from build123d import *

# Parameters (mm, degrees)
BOSS_EXTRUDE1_DEPTH = 21.59
SKETCH2_W           = 22.352
SKETCH2_H           = 21.6154
SKETCH2_R           = 3.175
BOSS_EXTRUDE2_DEPTH = 3.81
SKETCH3_R           = 3.175
BOSS_EXTRUDE3_DEPTH = 6.35
SKETCH4_W           = 27.94
SKETCH4_H           = 144.78
BOSS_EXTRUDE4_DEPTH = 48.388036719
SKETCH5_W           = 38.1
SKETCH5_H           = 30.48
SKETCH5_W_2         = 60.96
CUT_EXTRUDE1_DEPTH  = 385.104870976
SKETCH6_R           = 3.175
CUT_EXTRUDE2_DEPTH  = 833.884500924


with BuildPart() as part:
    # Sketch1 → Boss-Extrude1 (new body)
    with BuildSketch(Plane.XY):
        with BuildLine():
            Line((-792.583825879, 352.959436719), (-792.583825879, 356.769436719))
            Line((-792.583825879, 356.769436719), (-801.338321143, 356.769436719))
            ThreePointArc((-801.338321143, 356.769436719), (-803.772947911, 357.085841957), (-806.045825879, 358.014036719))
            ThreePointArc((-806.045825879, 358.014036719), (-810.863321143, 366.294436719), (-806.045825879, 374.574836719))
            Line((-806.045825879, 374.574836719), (-814.935825879, 374.574836719))
            Line((-814.935825879, 374.574836719), (-814.935825879, 352.959436719))
            Line((-814.935825879, 352.959436719), (-792.583825879, 352.959436719))
        make_face()
    extrude(amount=-BOSS_EXTRUDE1_DEPTH)

    # Sketch2 → Boss-Extrude2 (add)
    with BuildSketch(Plane.XY):
        with Locations((-803.759825879, 363.767136719)):
            Rectangle(SKETCH2_W, SKETCH2_H)
        with Locations(Location((-801.338321143, 366.294436719, 0), (0, 0, 180))):
            Circle(SKETCH2_R, mode=Mode.SUBTRACT)
    extrude(amount=BOSS_EXTRUDE2_DEPTH)

    # Sketch3 → Boss-Extrude3 (add)
    with BuildSketch(Plane(origin=(0, 0, -21.59), x_dir=(-1, 0, 0), z_dir=(0, 0, -1))):
        with BuildLine():
            Line((792.583825879, 356.769436719), (792.583825879, 374.574836719))
            Line((792.583825879, 374.574836719), (806.045825879, 374.574836719))
            ThreePointArc((806.045825879, 374.574836719), (810.546915906, 363.859809951), (801.338321143, 356.769436719))
            Line((801.338321143, 356.769436719), (792.583825879, 356.769436719))
        make_face()
        with Locations((801.338321143, 366.294436719)):
            Circle(SKETCH3_R, mode=Mode.SUBTRACT)
    extrude(amount=-BOSS_EXTRUDE3_DEPTH)

    # Sketch4 → Boss-Extrude4 (add)
    with BuildSketch(Plane.XZ.offset(-352.959436719)):
        with Locations((-813.665825879, 5.08)):
            Rectangle(SKETCH4_W, SKETCH4_H)
    extrude(amount=BOSS_EXTRUDE4_DEPTH)

    # Sketch5 → Cut-Extrude1 (cut, through all)
    with BuildSketch(Plane.ZY.offset(827.635825879)):
        with Locations((-48.26, 337.719436719)):
            Rectangle(SKETCH5_W, SKETCH5_H)
        with Locations((46.99, 337.719436719)):
            Rectangle(SKETCH5_W_2, SKETCH5_H)
    extrude(amount=-CUT_EXTRUDE1_DEPTH, mode=Mode.SUBTRACT)

    # Sketch6 → Cut-Extrude2 (cut, through all)
    with BuildSketch(Plane(origin=(0, 322.479436719, 0), x_dir=(1, 0, 0), z_dir=(0, 1, 0))):
        with Locations(Location((-820.039, 56.765714286, 0), (0, 0, 270))):
            Circle(SKETCH6_R)
        with Locations(Location((-820.039, -61.162857143, 0), (0, 0, 270))):
            Circle(SKETCH6_R)
    extrude(amount=-CUT_EXTRUDE2_DEPTH, mode=Mode.SUBTRACT)


solid = part.part
Geometry: final body of the model. Coordinates: model frame, mm. A direction names the side the tool comes from. Give positions to 0.01 mm unless a question says otherwise; leave off trailing zeros. Write each loop counter-clockwise with the first axis right and the second up, starting at its lowest first coordinate (ties: lowest second). Pieces come first, ordered by that corner, then holes. Notation, with made-up numbers: (-12, 33) - (32, 33) arc R36 cw to (32, 70) - close; hole circle Ø4 at (17.25, 55). An arc over 180 degrees is marked (long way). Return JSON: item names as keys, results as strings. Group by question number.
1) Section A-A on z = -55. Return the cut outline in (x, y), plus the area to 3 significant figures.
2) Mould query, pull axis X, two halves, no side actions, for faces 1 (the flat face through (-814.936, 364, -9)), 2 (the flat face through (-797, 356.769, -8)), 3 (the cylindrical face through (-804.367, 365.341, 1.878)). Classes: released by +X, released by -X, zero draft, split by the parting line, or undercut.
3) First-contact query: P1, Ø3.5, axis at x = -797.5, z = -4.5, coming from the -Y side; P2, Ø11, axis at x = -800, y = 368, coming from the -Z side; P3, Ø11, axis at y = 366, z = -3.5, coming from the -X side; P4, Ø3, axis at x = -797, y = 327.5, coming from the -Z side. Flat tips, straight axial feed; report the tip coordinate or a pass-through.
4) Section C-C on z = -18.5. Return the cut outline in (x, y) (3 decimals), plus the area to 3 significant figures.
5) Line query: line 1 (Z direction, x = -798.5, y = 363); line 2 (Y direction, x = -814, z = -38); line 3 (Z direction, x = -810, y = 343.5). Output: solid intervals per line, ascending.
6) Section D-D on z = -2.5. Return the cut outline in (x, y) (3 decimals), plus the area to 3 significant figures.
7) Section B-B on x = -812.5. Return the cut outline in (y, z), plus the area to 3 significant figures.
8) Set-up query: faces 4 (the flat face through (-804, 364, -21.59)), 5 (the flat face through (-798, 366, -15.24)), 6 (the flat face through (-804, 364, 3.81)), 7 (the flat face through (-814, 314, -67.31)). Return all of +Z, -Z, +X, -X, +Y, -Y with unobstructed straight access to the full face (end or side cutting, diameter ignored); none if empty.
Filled in:
{
 "1": {"outline": "(-827.64, 304.57) - (-822.68, 304.57) - (-822.68, 322.48) - (-827.64, 322.48) - close; (-817.4, 304.57) - (-799.7, 304.57) - (-799.7, 322.48) - (-817.4, 322.48) - close", "area": "406 mm^2"},
 "2": {"face 1": "released by -X", "face 2": "zero draft", "face 3": "undercut"},
 "3": {"P1": "stops at y = 352.96", "P2": "stops at z = -21.59", "P3": "stops at x = -814.94", "P4": "passes through"},
 "4": {"outline": "(-827.636, 304.571) - (-799.696, 304.571) - (-799.696, 352.959) - (-792.584, 352.959) - (-792.584, 374.575) - (-814.936, 374.575) - (-814.936, 352.959) - (-827.636, 352.959) - close; hole circle Ø6.35 at (-801.338, 366.294)", "area": "1,800 mm^2"},
 "5": {"line 1": "z = -21.59 to -15.24, 0 to 3.81", "line 2": "y = 304.57 to 322.48", "line 3": "z = -29.21 to 16.51"},
 "6": {"outline": "(-827.636, 304.571) - (-799.696, 304.571) - (-799.696, 352.959) - (-792.584, 352.959) - (-792.584, 356.769) - (-801.338, 356.769) arc R9.525 cw to (-806.046, 374.575) - (-814.936, 374.575) - (-814.936, 352.959) - (-827.636, 352.959) - close", "area": "1,540 mm^2"},
 "7": {"outline": "(304.57, -67.31) - (322.48, -67.31) - (322.48, -29.21) - (352.96, -29.21) - (352.96, -21.59) - (374.57, -21.59) - (374.57, 3.81) - (352.96, 3.81) - (352.96, 16.51) - (322.48, 16.51) - (322.48, 77.47) - (304.57, 77.47) - close", "area": "4,540 mm^2"},
 "8": {"face 4": "-Z, +X, -X, +Y", "face 5": "+X", "face 6": "+Z, +X, -X, +Y", "face 7": "-Z, +X, -X, +Y, -Y"}
}
